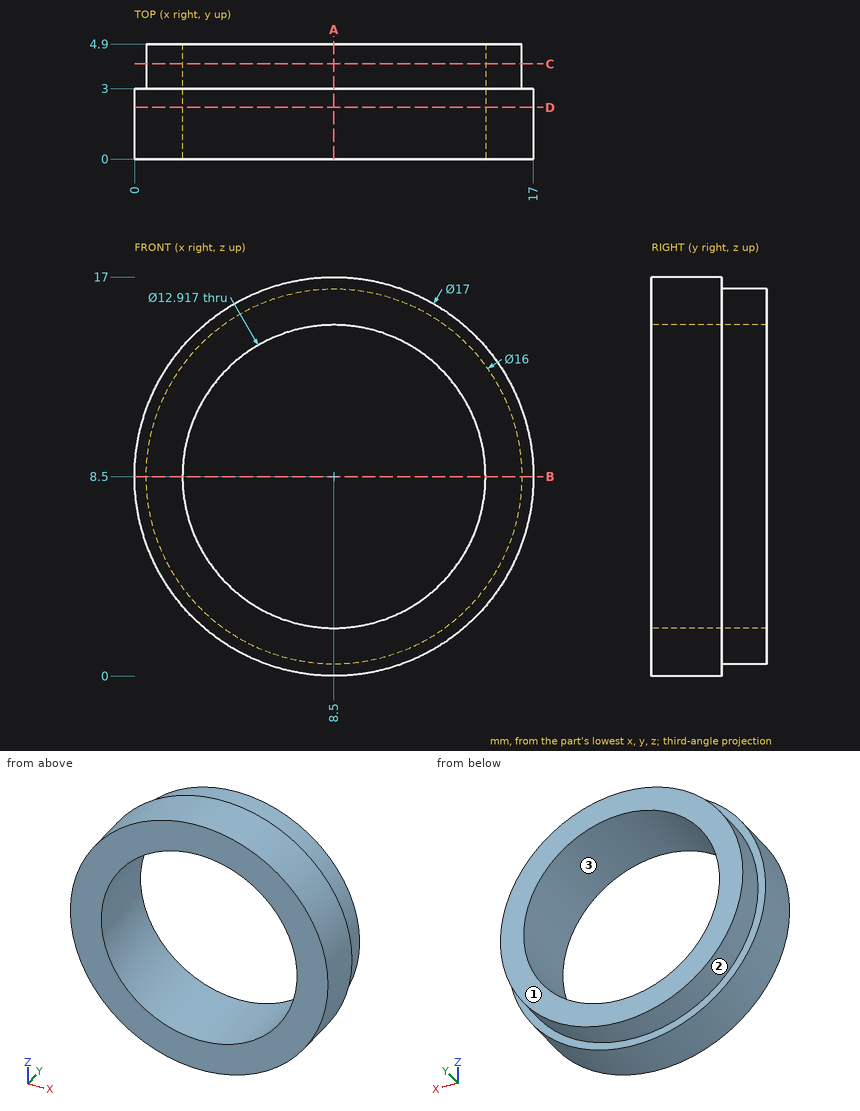
Here's the drawing with two shaded views (mm, measured from the low corner). I have some questions. Give positions to 0.01 mm unless a question says otherwise; leave off trailing zeros. Loops run counter-clockwise (first coordinate to the right, second up) from the corner with the lowest first, then second, coordinate; pieces in that order, holes last. Notation, with made-up numbers: M 55,42 L 114,42 A32 cw 114,78 Z; hole C 61,46.25 d7. An arc over 180 degrees is marked long. Use one line per item in the form item = value. Start each with the question number.
Q1. If we section it at C-C (y = 4.05): Write out the boundary of the cut face in (x, z), then the cut area to 3 significant figures.
Q2. If we section it at B-B (z = 8.5): Write out the boundary of the cut face in (x, y).
Q3. Thinking about a two-plate mould opening in Z: for the marked faces 1, 2 and 3, which applies, +Z half, -Z half, draft (parallel to the pull), parting line (faces both ways), or undercut?
Q4. If we section it at A-A (x = 8.5): Write out the boundary of the cut face in (y, z), then the cut area to 3 significant figures.
Q5. If we section it at D-D (y = 2.2): Write out the boundary of the cut face in (x, z), then the cut area to 3 significant figures.
Q6. I need wall thicknesses on line 1 along X through (y, z) = (2.6, 8.25); line 2 along X through (y, z) = (3.95, 8.5); line 3 along Z through (x, y) = (8.5, 2.55). Which ranges of each line are inside material? Lowest first, please.
Taken from the geometry:
q1.outline = C 8.5,8.5 d16; hole C 8.5,8.5 d12.92
q1.area = 70.0 mm^2
q2.outline = M 0,0 L 2.04,0 L 2.04,4.9 L 0.5,4.9 L 0.5,3 L 0,3 Z; M 14.96,0 L 17,0 L 17,3 L 16.5,3 L 16.5,4.9 L 14.96,4.9 Z
q3.face_1 = draft
q3.face_2 = parting line
q3.face_3 = undercut
q4.outline = M 0,0 L 3,0 L 3,0.5 L 4.9,0.5 L 4.9,2.04 L 0,2.04 Z; M 0,14.96 L 4.9,14.96 L 4.9,16.5 L 3,16.5 L 3,17 L 0,17 Z
q4.area = 18.1 mm^2
q5.outline = C 8.5,8.5 d17; hole C 8.5,8.5 d12.92
q5.area = 95.9 mm^2
q6.line_1 = 0 to 2.05, 14.95 to 17
q6.line_2 = 0.5 to 2.04, 14.96 to 16.5
q6.line_3 = 0 to 2.04, 14.96 to 17
